from build123d import *

# Parameters (mm, degrees)
SKETCH_1_W          = 73.6
SKETCH_1_H          = 58.5
EXTRUDE_1_DEPTH     = 22
CUT_EXTRUDE_2_DEPTH = 20
SKETCH_4_W          = 2
SKETCH_4_H          = 10.2
SKETCH_4_H_2        = 13.2
EXTRUDE_2_DEPTH     = 5


with BuildPart() as part:
    # Эскиз1 → Бобышка-Вытянуть1 (new body)
    with BuildSketch(Plane(origin=(0, 0, 0), x_dir=(1, 0, 0), z_dir=(0, 1, 0))):
        with Locations((36.8, -29.25)):
            Rectangle(SKETCH_1_W, SKETCH_1_H)
    extrude(amount=EXTRUDE_1_DEPTH)

    # Эскиз3 → Вырез-Вытянуть2 (cut)
    with BuildSketch(Plane(origin=(0, 22, 0), x_dir=(1, 0, 0), z_dir=(0, 1, 0))):
        Polygon((1.5, -1.8), (71.6, -1.8), (71.6, -5.3), (73.6, -5.3), (73.6, -15.5), (71.6, -15.5), (71.6, -34), (73.6, -34), (73.6, -47.2), (71.6, -47.2), (71.6, -56.7), (4.5, -56.7), (4.5, -45.5), (1.5, -45.5), align=None)
    extrude(amount=-CUT_EXTRUDE_2_DEPTH, mode=Mode.SUBTRACT)

    # Эскиз4 → Бобышка-Вытянуть2 (add)
    with BuildSketch(Plane(origin=(0, 2, 0), x_dir=(1, 0, 0), z_dir=(0, 1, 0))):
        with Locations((72.6, -10.4)):
            Rectangle(SKETCH_4_W, SKETCH_4_H)
        with Locations((72.6, -40.6)):
            Rectangle(SKETCH_4_W, SKETCH_4_H_2)
    extrude(amount=EXTRUDE_2_DEPTH)


solid = part.part
Check sheet for the modelled part. Datum: model origin and axes. Units: mm. A direction names the side the tool comes from. Round coordinates to 2 decimals unless told otherwise and drop trailing zeros. Loops run counter-clockwise (first coordinate to the right, second up) from the corner with the lowest first, then second, coordinate; pieces in that order, holes last. Notation, with made-up numbers: (-15.5, 82.5) - (15.5, 82.5) arc R32 cw to (15.5, 114.5) - close; hole circle Ø4 at (-5.5, 61.25). An arc over 180 degrees is marked (long way). Answer as CSV lines item,"result". Start each with the question number.
Item 1: Section check C-C (x = 36). Record the boundary of the cut face in (y, z).
Item 2: Section check B-B (z = 48.5). Record the boundary of the cut face in (x, y), and give its area (3 significant figures).
Item 3: Section check A-A (y = 8.25). Record the boundary of the cut face in (x, z), and give its area (3 significant figures).
Item 4: Release check for a two-part mould opening along X. For faces 4 (the flat face through (4.5, 12, 51)), 5 (the flat face through (73, 15, 34)), 6 (the flat face through (73.6, 11, 30)) record: +X half, -X half, draft (parallel to the pull), parting line (faces both ways), or undercut.
Item 5: Scan lines: line 1 (X direction, y = 19, z = 22.5); line 2 (Z direction, x = 51.5, y = 15.5); line 3 (Y direction, x = 57, z = 4). Record each from-to range of solid material in increasing order. Write a range as [from, to].
Item 6: Depth check by flat-ended pin: P1, Ø1, axis at x = 73, z = 40, coming from the +Y side. Enter the tip coordinate at first touch or a pass-through.
Item 7: Set-up check for faces 1 (the flat face through (73, 15, 15.5)), 2 (the flat face through (1.5, 12, 24)), 3 (the flat face through (1, 22, 31)): record each of +Z, -Z, +X, -X, +Y, -Y from which the full face is reachable in a straight line by a thin tool's end or side.
Report:
1,outline,"(0, 0) - (22, 0) - (22, 1.8) - (2, 1.8) - (2, 56.7) - (22, 56.7) - (22, 58.5) - (0, 58.5) - close"
2,outline,"(0, 0) - (73.6, 0) - (73.6, 22) - (71.6, 22) - (71.6, 2) - (4.5, 2) - (4.5, 22) - (0, 22) - close"
2,area,"277 mm2"
3,outline,"(0, 0) - (73.6, 0) - (73.6, 5.3) - (71.6, 5.3) - (71.6, 1.8) - (1.5, 1.8) - (1.5, 45.5) - (4.5, 45.5) - (4.5, 56.7) - (71.6, 56.7) - (71.6, 47.2) - (73.6, 47.2) - (73.6, 58.5) - (0, 58.5) - close; (71.6, 15.5) - (73.6, 15.5) - (73.6, 34) - (71.6, 34) - close"
3,area,"444 mm2"
4,face 4,"undercut"
4,face 5,"draft"
4,face 6,"+X half"
5,line 1,"x = [0, 1.5], [71.6, 73.6]"
5,line 2,"z = [0, 1.8], [56.7, 58.5]"
5,line 3,"y = [0, 2]"
6,P1,"stops at y = 7"
7,face 1,"+X, +Y"
7,face 2,"+Y"
7,face 3,"+Z, -Z, +X, -X, +Y"
